Input: part model. Units: mm. Frame: model coordinates. A direction names the side the tool comes from. Give positions to 0.01 mm unless a question says otherwise; leave off trailing zeros. Loops run counter-clockwise (first coordinate to the right, second up) from the corner with the lowest first, then second, coordinate; pieces in that order, holes last. Notation, with made-up numbers: M 56,-5.5 L 94,-5.5 A19 cw 94,1.5 Z; hole C 1.5,37 d2. An arc over 180 degrees is marked long. Answer as a JSON object with one key per item and string values. Group by question number.
1) Section query C-C on x = -20. Return loops of the section in (y, z) (3 decimals).
2) Section query D-D on x = 7. Return loops of the section in (y, z), plus the area to 3 significant figures.
3) Section query A-A on x = 54. Return loops of the section in (y, z).
4) Draft query along X for faces 5 (the flat face through (-60, 29, 4)), 6 (the cylindrical face through (19.48, 29.6, 0.99)), 7 (the flat face through (-1, 32, 7)), 8 (the cylindrical face through (-20.43, 23.68, 4.46)). Return one class per face: +X half, -X half, draft (parallel to the pull), parting line (faces both ways), or undercut.
5) Ray query, L1, parallel to X at y = 16.27, z = 5.9; L2, parallel to X at y = 20.5, z = 3; L3, parallel to X at y = 26.75, z = 1.75. Return the intervals inside material, ascending.
6) Access query for faces 1 (the flat face through (12.5, 20, 4)), 2 (the flat face through (54, 19, 5)), 3 (the cylindrical face through (-22.948, 28.338, 0.986)), 4 (the flat face through (-54, 19, 5)). Directions: +Z, -Z, +X, -X, +Y, -Y. A direction counts if a zero-diameter tool reaches every point of the face in a straight line with its end or side. Return the directions, or none.
7) Section query B-B on y = 16.27. Return loops of the section in (x, z).
8) First-contact query: P1, Ø9, axis at x = -19.5, y = 25, coming from the -Z side; P2, Ø5, axis at x = -20, y = 25.635, coming from the -Z side; P3, Ø6, axis at x = -52, y = 16.5, coming from the -Z side; P4, Ø3, axis at x = -8, z = 4.5, coming from the -Y side. Flat tips, straight axial feed; report the tip coordinate or a pass-through.
from build123d import *

# Parameters (mm, degrees)
SKETCH2_W           = 120
SKETCH2_H           = 28.73
SKETCH2_R           = 1.5
SKETCH2_R_2         = 2
BOSS_EXTRUDE1_DEPTH = 7
SKETCH3_W           = 12
SKETCH3_H           = 13.95
CUT_EXTRUDE1_DEPTH  = 5
SKETCH4_W           = 25
SKETCH4_H           = 46.747057702
CUT_EXTRUDE2_DEPTH  = 7
SKETCH5_R           = 4
CUT_EXTRUDE3_DEPTH  = 2


with BuildPart() as part:
    # Sketch2 → Boss-Extrude1 (new body)
    with BuildSketch(Plane.XY):
        with Locations((0, 25.635)):
            Rectangle(SKETCH2_W, SKETCH2_H)
        with Locations((-54, 16.27)):
            Circle(SKETCH2_R, mode=Mode.SUBTRACT)
        with Locations((54, 16.27)):
            Circle(SKETCH2_R, mode=Mode.SUBTRACT)
        with Locations((-20, 25.635)):
            Circle(SKETCH2_R_2, mode=Mode.SUBTRACT)
        with Locations(Location((20, 25.635, 0), (0, 0, 180))):
            Circle(SKETCH2_R_2, mode=Mode.SUBTRACT)
    extrude(amount=BOSS_EXTRUDE1_DEPTH)

    # Sketch3 → Cut-Extrude1 (cut)
    with BuildSketch(Plane(origin=(0, 0, 0), x_dir=(-1, 0, 0), z_dir=(0, 0, -1))):
        with Locations((-54, 16.135)):
            Rectangle(SKETCH3_W, SKETCH3_H)
        with Locations((54, 16.135)):
            Rectangle(SKETCH3_W, SKETCH3_H)
    extrude(amount=-CUT_EXTRUDE1_DEPTH, mode=Mode.SUBTRACT)

    # Sketch4 → Cut-Extrude2 (cut)
    with BuildSketch(Plane.XY.offset(7)):
        with Locations((0, 5.58721862)):
            Rectangle(SKETCH4_W, SKETCH4_H)
    extrude(amount=-CUT_EXTRUDE2_DEPTH, mode=Mode.SUBTRACT)

    # Sketch5 → Cut-Extrude3 (cut)
    with BuildSketch(Plane.XY):
        with Locations((20, 25.635)):
            Circle(SKETCH5_R)
        with Locations((-20, 25.635)):
            Circle(SKETCH5_R)
    extrude(amount=CUT_EXTRUDE3_DEPTH, mode=Mode.SUBTRACT)


solid = part.part
Output:
{
 "1": {"outline": "M 11.27,0 L 21.635,0 L 21.635,2 L 23.635,2 L 23.635,7 L 11.27,7 Z; M 27.635,2 L 29.635,2 L 29.635,0 L 40,0 L 40,7 L 27.635,7 Z"},
 "2": {"outline": "M 28.96,0 L 40,0 L 40,7 L 28.96,7 Z", "area": "77.3 mm^2"},
 "3": {"outline": "M 11.27,5 L 14.77,5 L 14.77,7 L 11.27,7 Z; M 17.77,5 L 23.11,5 L 23.11,0 L 40,0 L 40,7 L 17.77,7 Z"},
 "4": {"face 5": "-X half", "face 6": "undercut", "face 7": "draft", "face 8": "undercut"},
 "5": {"L1": "x = -60 to -55.5, -52.5 to -12.5, 12.5 to 52.5, 55.5 to 60", "L2": "x = -48 to -12.5, 12.5 to 48", "L3": "x = -60 to -23.84, -16.16 to -12.5, 12.5 to 16.16, 23.84 to 60"},
 "6": {"face 1": "+Z, -Z, -Y", "face 2": "-Z, +X, -Y", "face 3": "-Z", "face 4": "-Z, -X, -Y"},
 "7": {"outline": "M -60,5 L -55.5,5 L -55.5,7 L -60,7 Z; M -52.5,5 L -48,5 L -48,0 L -12.5,0 L -12.5,7 L -52.5,7 Z; M 12.5,0 L 48,0 L 48,5 L 52.5,5 L 52.5,7 L 12.5,7 Z; M 55.5,5 L 60,5 L 60,7 L 55.5,7 Z"},
 "8": {"P1": "stops at z = 0", "P2": "stops at z = 2", "P3": "stops at z = 5", "P4": "stops at y = 28.96"}
}
